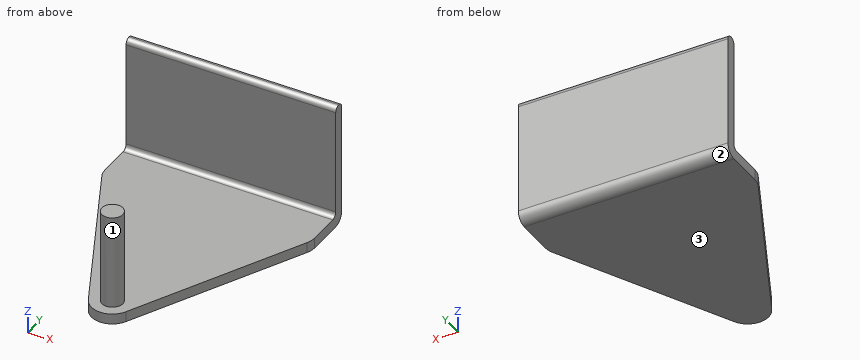
```python
from build123d import *

# Parameters (mm, degrees)
F0_W     = 200
F0_H     = 50
F1_DEPTH = 10
F2_R     = 20
F3_R     = 10
F4_DEPTH = 90
F5_W     = 200
F5_H     = 10
F6_DEPTH = 110
F7_R     = 4.99999
F8_R     = 10


# Not quite as in the source:
# - a fillet or chamfer is up to 0.001 mm smaller than in the source, because OpenCascade refuses the exact size


with BuildPart() as f1:
    # F0 (on Top) → F1 (new body)
    with BuildSketch(Plane.XY):
        Polygon((200, 0), (0, 0), (98.8994031925, -202.201193615), align=None)
        with Locations((100, 25)):
            Rectangle(F0_W, F0_H)
    extrude(amount=F1_DEPTH)

    # F2
    f2_edges = [f1.edges().sort_by_distance(p)[0] for p in [
        (98.899403, -202.201194, 5),
        (200, 0, 5),
        (0, 0, 5),
    ]]
    fillet(f2_edges, radius=F2_R)

    # F3 (on face) → F4 (join)
    with BuildSketch(Plane.XY.offset(10)):
        with Locations((99.0967144561, -157.0852115379)):
            Circle(F3_R)
    extrude(amount=F4_DEPTH)

    # F5 (on face) → F6 (join)
    with BuildSketch(Plane.XY.offset(10)):
        with Locations((100, 45)):
            Rectangle(F5_W, F5_H)
    extrude(amount=F6_DEPTH)

    # F7 (radius 5 in the source; OpenCascade refuses exactly that, so slightly less here)
    f7_edges = [f1.edges().sort_by_distance(p)[0] for p in [
        (100, 50, 120),
        (100, 40, 120),
        (100, 40, 10),
    ]]
    fillet(f7_edges, radius=F7_R)

    # F8
    f8_edges = [f1.edges().sort_by_distance(p)[0] for p in [
        (100, 50, 0),
    ]]
    fillet(f8_edges, radius=F8_R)


solid = f1.part
```
Check sheet for the modelled part. Datum: model origin and axes. Units: mm. Face numbers are marked on the shaded views. Round coordinates to 2 decimals unless told otherwise and drop trailing zeros. Order: outer loops, then holes, each group sorted by start corner. A loop starts at its lowest first (then second) coordinate and runs counter-clockwise, first axis right, second up. Notation, with made-up numbers: (21, -6) -> (53, -6) arc R12 ccw to (53, 13) -> close; hole circle Ø7 at (-12, 49). An arc over 180 degrees is marked (long way). One line per item, written item: value. Start each with the question number.
Q1. Mould release check, pull along Y, two halves, no side actions. Record for the marked faces 1, 2 and 3: pulls with the +Y half, pulls with the -Y half, needs draft (parallel to the pull), parting line crosses it, or undercut.
Q2. Gauge pin test, flat ends, axial feed: pin 1 Ø22 at (x, y) = (98.5, -159) entering from +Z; pin 2 Ø1.5 at (x, z) = (153.5, 33.5) entering from -Y. Record the tip position at first contact, or that the pin passes through.
Q3. Thickness scan on line 1 (Z direction, x = 38, y = -40); line 2 (Y direction, x = 171.5, z = 69); line 3 (Z direction, x = 47.5, y = 37.5). Record the ranges inside material, lowest first.
Q4. Cross-section at B-B (y = -162.5). Record the boundary of the cut face in (x, z).
Q5. Cross-section at C-C (z = 77). Record the boundary of the cut face in (x, y), and give its area (3 significant figures).
Completed:
1. face 1: undercut
1. face 2: pulls with the +Y half
1. face 3: needs draft
2. pin 1: stops at z = 100
2. pin 2: stops at y = 40
3. line 1: z = 0 to 10
3. line 2: y = 40 to 50
3. line 3: z = 0 to 10.67
4. outline: (79.48, 0) -> (118.75, 0) -> (118.75, 10) -> (107.5, 10) -> (107.5, 100) -> (90.69, 100) -> (90.69, 10) -> (79.48, 10) -> close
5. outline: (0, 40) -> (200, 40) -> (200, 50) -> (0, 50) -> close; circle Ø20 at (99.1, -157.09)
5. area: 2,310 mm²
